The model under review builds one solid part; all positions refer to its coordinate system, in mm. Face numbers are marked on the shaded views. A direction names the side the tool comes from. Give positions to 0.01 mm unless a question says otherwise; leave off trailing zeros. Order: outer loops, then holes, each group sorted by start corner. A loop starts at its lowest first (then second) coordinate and runs counter-clockwise, first axis right, second up. Notation, with made-up numbers: (67.5, 12) - (114.5, 12) arc R27 ccw to (114.5, 46) - close; hole circle Ø7 at (42.25, 85.5). An arc over 180 degrees is marked (long way). Use CSV: the item, a comma, the result in double quotes.
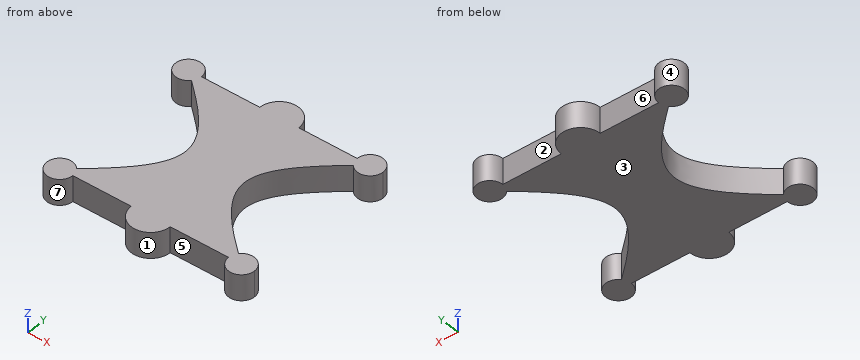
```python
from build123d import *

# Parameters (mm, degrees)
F1_DEPTH = 2


with BuildPart() as f1:
    # F0 (on Top) → F1 (new body)
    with BuildSketch(Plane.XY):
        with BuildLine():
            add(Edge.make_bspline(
                [(-6.237544, -0.64704), (-6.489718, -0.43136), (-6.744859, -0.21568), (-7, 0)],
                knots=[14.458679, 14.458679, 14.458679, 14.458679, 15.282723, 15.282723, 15.282723, 15.282723], degree=3))
            Line((-7, 0), (-6, 0))
            ThreePointArc((-6, 0), (-7.938738, 0.344633), (-6.237544, -0.64704))
        make_face()
        with BuildLine():
            Line((-6, 0), (-7, 0))
            add(Edge.make_bspline(
                [(-6.237544, -0.64704), (-6.489718, -0.43136), (-6.744859, -0.21568), (-7, 0)],
                knots=[14.458679, 14.458679, 14.458679, 14.458679, 15.282723, 15.282723, 15.282723, 15.282723], degree=3))
            ThreePointArc((-6.237544, -0.64704), (-6.061262, -0.344633), (-6, 0))
        make_face()
        with BuildLine():
            Line((-1.5, 0), (-6, 0))
            ThreePointArc((-6, 0), (-6.061262, -0.344633), (-6.237544, -0.64704))
            add(Edge.make_bspline(
                [(-2.26815, -6), (-2.26815, -4.21568), (-4.151307, -2.43136), (-6.237544, -0.64704)],
                knots=[7.641361, 7.641361, 7.641361, 7.641361, 14.458679, 14.458679, 14.458679, 14.458679], degree=3))
            Line((-2.26815, -6), (0, -6))
            Line((0, -6), (0, 0))
            Line((0, 0), (-1.5, 0))
        make_face()
        with BuildLine():
            ThreePointArc((1.5, 0), (0, 1.5), (-1.5, 0))
            Line((-1.5, 0), (0, 0))
            Line((0, 0), (1.5, 0))
        make_face()
        with BuildLine():
            Line((1.5, 0), (0, 0))
            Line((0, 0), (0, -6))
            Line((0, -6), (2.26815, -6))
            add(Edge.make_bspline(
                [(2.26815, -6), (2.26815, -4.21568), (4.151307, -2.43136), (6.237544, -0.64704)],
                knots=[7.641361, 7.641361, 7.641361, 7.641361, 14.458679, 14.458679, 14.458679, 14.458679], degree=3))
            ThreePointArc((6.237544, -0.64704), (6.061262, -0.344633), (6, 0))
            Line((6, 0), (1.5, 0))
        make_face()
        with BuildLine():
            Line((7, 0), (6, 0))
            ThreePointArc((6, 0), (6.061262, -0.344633), (6.237544, -0.64704))
            add(Edge.make_bspline(
                [(6.237544, -0.64704), (6.489718, -0.43136), (6.744859, -0.21568), (7, 0)],
                knots=[14.458679, 14.458679, 14.458679, 14.458679, 15.282723, 15.282723, 15.282723, 15.282723], degree=3))
        make_face()
        with BuildLine():
            ThreePointArc((8, 0), (7, 1), (6, 0))
            Line((6, 0), (7, 0))
            add(Edge.make_bspline(
                [(6.237544, -0.64704), (6.489718, -0.43136), (6.744859, -0.21568), (7, 0)],
                knots=[14.458679, 14.458679, 14.458679, 14.458679, 15.282723, 15.282723, 15.282723, 15.282723], degree=3))
            ThreePointArc((6.237544, -0.64704), (7.344633, -0.938738), (8, 0))
        make_face()
        with BuildLine():
            Line((0, -6), (-2.26815, -6))
            add(Edge.make_bspline(
                [(-6.237544, -11.35296), (-4.151307, -9.56864), (-2.26815, -7.78432), (-2.26815, -6)],
                knots=[0.824044, 0.824044, 0.824044, 0.824044, 7.641361, 7.641361, 7.641361, 7.641361], degree=3))
            ThreePointArc((-6.237544, -11.35296), (-6.061262, -11.655367), (-6, -12))
            Line((-6, -12), (-1.5, -12))
            Line((-1.5, -12), (0, -12))
            Line((0, -12), (0, -6))
        make_face()
        with BuildLine():
            Line((2.26815, -6), (0, -6))
            Line((0, -6), (0, -12))
            Line((0, -12), (1.5, -12))
            Line((1.5, -12), (6, -12))
            ThreePointArc((6, -12), (6.061262, -11.655367), (6.237544, -11.35296))
            add(Edge.make_bspline(
                [(6.237544, -11.35296), (4.151307, -9.56864), (2.26815, -7.78432), (2.26815, -6)],
                knots=[0.824044, 0.824044, 0.824044, 0.824044, 7.641361, 7.641361, 7.641361, 7.641361], degree=3))
        make_face()
        with BuildLine():
            ThreePointArc((-6, -12), (-6.061262, -11.655367), (-6.237544, -11.35296))
            add(Edge.make_bspline(
                [(-7, -12), (-6.744859, -11.78432), (-6.489718, -11.56864), (-6.237544, -11.35296)],
                knots=[0, 0, 0, 0, 0.824044, 0.824044, 0.824044, 0.824044], degree=3))
            Line((-7, -12), (-6, -12))
        make_face()
        with BuildLine():
            add(Edge.make_bspline(
                [(-7, -12), (-6.744859, -11.78432), (-6.489718, -11.56864), (-6.237544, -11.35296)],
                knots=[0, 0, 0, 0, 0.824044, 0.824044, 0.824044, 0.824044], degree=3))
            ThreePointArc((-6.237544, -11.35296), (-7.938738, -12.344633), (-6, -12))
            Line((-6, -12), (-7, -12))
        make_face()
        with BuildLine():
            Line((1.5, -12), (0, -12))
            Line((0, -12), (-1.5, -12))
            ThreePointArc((-1.5, -12), (0, -13.5), (1.5, -12))
        make_face()
        with BuildLine():
            add(Edge.make_bspline(
                [(7, -12), (6.744859, -11.78432), (6.489718, -11.56864), (6.237544, -11.35296)],
                knots=[0, 0, 0, 0, 0.824044, 0.824044, 0.824044, 0.824044], degree=3))
            ThreePointArc((6.237544, -11.35296), (6.061262, -11.655367), (6, -12))
            Line((6, -12), (7, -12))
        make_face()
        with BuildLine():
            ThreePointArc((8, -12), (7.344633, -11.061262), (6.237544, -11.35296))
            add(Edge.make_bspline(
                [(7, -12), (6.744859, -11.78432), (6.489718, -11.56864), (6.237544, -11.35296)],
                knots=[0, 0, 0, 0, 0.824044, 0.824044, 0.824044, 0.824044], degree=3))
            Line((7, -12), (6, -12))
            ThreePointArc((6, -12), (7, -13), (8, -12))
        make_face()
    extrude(amount=F1_DEPTH)


solid = f1.part
```
Item 1: Tool access review of the marked faces 5, 6 and 7: name each direction out of +Z, -Z, +X, -X, +Y, -Y from which nothing blocks a thin tool from reaching the whole face with its end or side.
Results list:
face 5,"+Z, -Z, -Y"
face 6,"+Z, -Z, +Y"
face 7,"+Z, -Z"
Item 2: Wall thickness on L1, parallel to Y at x = 7, z = 0.55; L2, parallel to Y at x = -6.5, z = 0.7; L3, parallel to Y at x = -2, z = 0.65: over which ranges is each line inside the solid? List them lowest first.
Results list:
L1,"y = -13 to -11, -1 to 1"
L2,"y = -12.87 to -11.13, -0.87 to 0.87"
L3,"y = -12 to 0"
Item 3: Mouldability with a two-part tool opening along Y and no side actions: class the marked faces 1, 2, 3 and 4 as pulls with the +Y half, pulls with the -Y half, needs draft (parallel to the pull), parting line crosses it, or undercut.
Results list:
face 1,"pulls with the -Y half"
face 2,"pulls with the +Y half"
face 3,"needs draft"
face 4,"undercut"
Item 4: Clearance check with a flat-ended pin moving along its axis: pin 1 (2 mm diameter, centred on x = 1, y = -1, fed in from -Z). State where the tip first meets the part, or that it passes through.
Results list:
pin 1,"stops at z = 0"
Item 5: Take a section at B-B, the plane x = 2. Give the boundary of the cut face in (y, z), and give its area (3 significant figures).
Results list:
outline,"(-12, 0) - (0, 0) - (0, 2) - (-12, 2) - close"
area,"24.0 mm2"
Item 6: Take a section at A-A, the plane x = 7. Give the boundary of the cut face in (y, z), and give its area (3 significant figures).
Results list:
outline,"(-13, 0) - (-11, 0) - (-11, 2) - (-13, 2) - close; (-1, 0) - (1, 0) - (1, 2) - (-1, 2) - close"
area,"8.00 mm2"
